Input: part model. Units: mm. Frame: model coordinates. Coordinates: 2 decimals unless noted, no trailing zeros. Loops run counter-clockwise (first coordinate to the right, second up) from the corner with the lowest first, then second, coordinate; pieces in that order, holes last.
Autodesk Inventor part; units mm, degrees
ref_plane "YZ Plane" through (0, 0, 0) normal (1, 0, 0) x (0, 1, 0)
ref_plane "XZ Plane" through (0, 0, 0) normal (0, 1, 0) x (-1, 0, 0)
ref_plane "XY Plane" through (0, 0, 0) normal (0, 0, 1) x (1, 0, 0)
sketch "Sketch1" plane through (0, 0, 0) normal (0, 0, 1) x (1, 0, 0)
  circle A0 centre (0, 0) radius 6.5
  line L0 (6.5, 0) -> (6.35, 0)
  line L1 (6.35, 0) -> (6.35, 11)
  line L2 (6.35, 11) -> (6.5, 11)
  line L3 (6.5, 11) -> (6.5, 0)
  circle A1 centre (0, 0) radius 5.3
  point P0 (6.35, 1.3883)
  dimension "d0" = 13
  dimension "d1" = 0.15
  dimension "d2" = 11
  dimension "d12" = 1.2
extrude "Extrusion1" add sketch "Sketch1" along normal blind 8.46
sketch "Sketch2" plane through (6.5, 0, 0) normal (1, 0, 0) x (0, 0, -1)
  circle A0 centre (-4.23, 5) radius 1.61
  line L0 (0, 0) -> (0, 11)
  line L1 (-8.46, 0) -> (-8.46, 11)
  arc A1 (0, 9.3706) -> (-8.46, 9.3706) centre (-4.23, 4.8377) ccw
  line L2 (-8.46, 0) -> (0, 0)
  line L3 (0, 6.5) -> (0, -6.5)
  line L4 (0, 0) -> (0, 11)
  line L5 (0, 11) -> (-8.46, 11)
  line L6 (-8.46, 0) -> (-8.46, 11)
  line L7 (0, 0) -> (-8.46, 0)
  point P0 (0, 1.3883)
  point P1 (-3.5473, 11)
  point P2 (-4.9127, 11)
  dimension "d5" = 5
  dimension "d6" = 3.22
  dimension "d8" = 4.23
  dimension "d9" = 6.2
extrude "Extrusion2" cut sketch "Sketch2" against normal up to surface (0.15 mm away) contours A0 | A1 L5 L0 | L1 L5 A1
properties part number "LCF 025 05 031S (on hub)" material "Brass, Soft Yellow"
Item 1: Section query C-C (y = 2). Output: boundary loops of the cut face in (x, z), then the cut area to 3 significant figures.
Result:
outline: (-6.18, 0) - (-4.91, 0) - (-4.91, 8.46) - (-6.18, 8.46) - close; (4.91, 0) - (6.18, 0) - (6.18, 8.46) - (4.91, 8.46) - close; (6.35, 0) - (6.5, 0) - (6.5, 8.46) - (6.35, 8.46) - close
area: 22.9 mm2
Item 2: Mould query, pull axis X, two halves, no side actions, for faces 1 (the face through (-4, -4, 8.46)), 2 (the face through (6.5, 7, 4)), 3 (the face through (-6.427, -0.972, 4.171)). Classes: +X half, -X half, draft (parallel to the pull), parting line (faces both ways), or undercut.
Result:
face 1: draft
face 2: +X half
face 3: undercut
Item 3: Contact query for flat-ended pins moving along their axis: P1, Ø4, axis at y = 3, z = 4.5, coming from the -X side; P2, Ø3, axis at y = 6.5, z = 4.5, coming from the -X side; P3, Ø1.5, axis at y = -3, z = 5, coming from the +X side. Output: stop coordinate, or through.
Result:
P1: stops at x = -6.42
P2: stops at x = -4.15
P3: stops at x = 6.1
Item 4: Section query A-A (z = 4.23). Output: boundary loops of the cut face in (x, y).
Result:
outline: (6.35, 1.39) arc R6.5 ccw (long way) to (6.5, 0) - (6.5, 3.39) - (6.35, 3.39) - close; (6.35, 6.61) - (6.5, 6.61) - (6.5, 11) - (6.35, 11) - close; hole circle Ø10.6 at (0, 0)
Item 5: Section query B-B (x = 0). Output: boundary loops of the cut face in (y, z).
Result:
outline: (-6.5, 0) - (-5.3, 0) - (-5.3, 8.46) - (-6.5, 8.46) - close; (5.3, 0) - (6.5, 0) - (6.5, 8.46) - (5.3, 8.46) - close
Item 6: Section query D-D (z = 5.5). Output: boundary loops of the cut face in (x, y), then the cut area to 3 significant figures.
Result:
outline: (6.35, 1.39) arc R6.5 ccw (long way) to (6.5, 0) - (6.5, 4.01) - (6.35, 4.01) - close; (6.35, 5.99) - (6.5, 5.99) - (6.5, 10.91) - (6.35, 10.91) - close; hole circle Ø10.6 at (0, 0)
area: 45.7 mm2
Item 7: Line query: L1, parallel to Y at x = 0, z = 6.5; L2, parallel to X at y = -0.25, z = 4.5; L3, parallel to X at y = -1, z = 7. Output: solid intervals per line, ascending.
Result:
L1: y = -6.5 to -5.3, 5.3 to 6.5
L2: x = -6.5 to -5.29, 5.29 to 6.5
L3: x = -6.42 to -5.2, 5.2 to 6.42
